Source: CAD feature listing. Evaluate the final solid. Frame: model axes, mm. A direction names the side the tool comes from. Coordinates: 2 decimals unless noted, no trailing zeros. Write each loop counter-clockwise with the first axis right and the second up, starting at its lowest first coordinate (ties: lowest second). Pieces come first, ordered by that corner, then holes. Notation, with made-up numbers: (37, 17) -> (86, 17) arc R30 ccw to (86, 50) -> close; hole circle Ø7 at (75, 43.5). An arc over 180 degrees is marked (long way). One line per item, written item: value. Start each with the question number.
1. Access query for faces 1 (the flat face through (25, 7, 0)), 2 (the cylindrical face through (46.99, -2.46, -62.15)). Directions: +Z, -Z, +X, -X, +Y, -Y. A direction counts if a zero-diameter tool reaches every point of the face in a straight line with its end or side. Return the directions, or none.
2. Section query C-C, the plane z = -3. Output: boundary loops of the cut face in (x, y), and give its area (3 significant figures).
3. Section query D-D, the plane x = 12.5. Output: boundary loops of the cut face in (y, z).
4. Section query A-A, the plane z = -45. Output: boundary loops of the cut face in (x, y), and give its area (3 significant figures).
5. Section query B-B, the plane x = 25. Output: boundary loops of the cut face in (y, z), and give its area (3 significant figures).
6. Line query: line 1 (Z direction, x = 25, y = -1.55); line 2 (Z direction, x = 40.5, y = 5.25); line 3 (Y direction, x = 16, z = -18.5). Output: solid intervals per line, ascending.
7. First-contact query: P1, Ø15, axis at x = 18.5, z = -16.5, coming from the +Y side; P2, Ø7.5, axis at x = 23.5, y = 5, coming from the -Z side. Flat tips, straight axial feed; report the tip coordinate or a pass-through.
8. Mould query, pull axis Z, two halves, no side actions, for faces 3 (the flat face through (0, -1, -18)), 4 (the cylindrical face through (24.09, -2.54, -38.06)), 5 (the flat face through (25, 5, 5)). Classes: released by +Z, released by -Z, zero draft, split by the parting line, or undercut.
from build123d import *

# Parameters (mm, degrees)
F1_DEPTH = 50
F2_R     = 7
F3_DEPTH = 25
F4_R     = 10


with BuildPart() as f1:
    # F0 (on Right) → F1 (new body)
    with BuildSketch(Plane.YZ):
        Polygon((-5, -65), (0, -65), (0, 0), (15, 0), (15, 5), (-5, 5), align=None)
    extrude(amount=F1_DEPTH)

    # F2 (on face) → F3 (cut)
    with BuildSketch(Plane.XZ.offset(5)):
        with Locations((25, -45)):
            Circle(F2_R)
    extrude(amount=-F3_DEPTH, mode=Mode.SUBTRACT)

    # F4
    f4_edges = [f1.edges().sort_by_distance(p)[0] for p in [
        (0, -2.5, -65),
        (50, -2.5, -65),
    ]]
    fillet(f4_edges, radius=F4_R)


solid = f1.part
Computed values:
1. face 1: -Z, +X, -X, +Y
1. face 2: -Z, +X, +Y, -Y
2. outline: (0, -5) -> (50, -5) -> (50, 0) -> (0, 0) -> close
2. area: 250 mm²
3. outline: (-5, -65) -> (0, -65) -> (0, 0) -> (15, 0) -> (15, 5) -> (-5, 5) -> close
4. outline: (0, -5) -> (18, -5) -> (18, 0) -> (0, 0) -> close; (32, -5) -> (50, -5) -> (50, 0) -> (32, 0) -> close
4. area: 180 mm²
5. outline: (-5, -65) -> (0, -65) -> (0, -52) -> (-5, -52) -> close; (-5, -38) -> (0, -38) -> (0, 0) -> (15, 0) -> (15, 5) -> (-5, 5) -> close
5. area: 355 mm²
6. line 1: z = -65 to -52, -38 to 5
6. line 2: z = 0 to 5
6. line 3: y = -5 to 0
7. P1: stops at y = 0
7. P2: stops at z = 0
8. face 3: zero draft
8. face 4: undercut
8. face 5: released by +Z
